Check sheet for the modelled part. Datum: model origin and axes. Units: mm. A direction names the side the tool comes from. Round coordinates to 2 decimals unless told otherwise and drop trailing zeros. Loops run counter-clockwise (first coordinate to the right, second up) from the corner with the lowest first, then second, coordinate; pieces in that order, holes last. Notation, with made-up numbers: M 1,-31 L 29,-31 A25 cw 29,4 Z; hole C -36,-6.75 d1. An arc over 180 degrees is marked long. One line per question, with ' | ' between items. Start each with the question number.
(1) Section check A-A (y = 0). Record the boundary of the cut face in (x, z).
(2) Tool access check on faces 4 (the face through (-1, 2, 0)), 5 (the face through (-0.54, 2.44, 5.42)). Record the directions out of +Z, -Z, +X, -X, +Y, -Y that give a thin tool (end or side, any length) a straight path to the whole face; none if there is none.
(3) Section check D-D (y = 2.25). Record the boundary of the cut face in (x, z).
(4) Section check C-C (z = 9). Record the boundary of the cut face in (x, y).
(5) Go/stop test with flat-tipped pins: P1, Ø4, axis at x = 2, y = 2, coming from the -Z side; P2, Ø1, axis at x = 1, z = 1.5, coming from the +Y side. Record where each tip stops, or that it passes through.
(6) Thickness scan on probe 1 along Y at (x, z) = (0, 4.75); probe 2 along Z at (x, y) = (-1.25, -3.25); probe 3 along X at (y, z) = (-0.75, 2.5). Record the ranges inside material, lowest first. Write a range as [from, to].
(7) Draft check along X on faces 1 (the face through (2, 2, 11)), 2 (the face through (-0.867, -3.905, 11.507)), 3 (the face through (-1.5, -0.07, 5.92)). Enter one of: +X half, -X half, draft (parallel to the pull), parting line (faces both ways), or undercut.
Autodesk Inventor part; units mm, degrees
ref_plane "YZ Plane" through (0, 0, 0) normal (1, 0, 0) x (0, 1, 0)
ref_plane "XZ Plane" through (0, 0, 0) normal (0, 1, 0) x (-1, 0, 0)
ref_plane "XY Plane" through (0, 0, 0) normal (0, 0, 1) x (1, 0, 0)
sketch "Skizze1" plane through (0, 0, 0) normal (0, 0, 1) x (1, 0, 0)
  circle A0 centre (0, 0) radius 2.5
  circle A1 centre (0, 0) radius 1.5
  dimension "d0" = 1
  dimension "d1" = 5
extrude "Extrusion1" add sketch "Skizze1" along normal blind 12
chamfer "Fase1" distance 0.5 angle 45 2 edges at (-1.5, 0, 12) (-1.5, 0, 0)
sketch "Skizze2" plane through (0, 0, 12) normal (0, 0, 1) x (1, 0, 0)
  circle A0 centre (0, 0) radius 2.5
  circle A1 centre (0, 0) radius 2
  circle A2 centre (0, 0) radius 4
  dimension "d7" = 8
extrude "Extrusion2" add sketch "Skizze2" against normal blind 1 contours A2
properties part number "13_0204_048"
The answers:
1) outline: M -4,11 L -2.5,11 L -2.5,0 L -2,0 L -1.5,0.5 L -1.5,11.5 L -2,12 L -4,12 Z; M 1.5,0.5 L 2,0 L 2.5,0 L 2.5,11 L 4,11 L 4,12 L 2,12 L 1.5,11.5 Z
2) face 4: -Z, +X, -X, +Y, -Y | face 5: -Z
3) outline: M -3.31,11 L -1.09,11 L -1.09,0 L 1.09,0 L 1.09,11 L 3.31,11 L 3.31,12 L -3.31,12 Z
4) outline: C 0,0 d5; hole C 0,0 d3
5) P1: z = 0 | P2: y = 2.45
6) probe 1: [-2.5, -1.5], [1.5, 2.5] | probe 2: [11, 12] | probe 3: [-2.38, -1.3], [1.3, 2.38]
7) face 1: draft | face 2: parting line | face 3: undercut
